```python
from build123d import *

# Parameters (mm, degrees)
EXTRUDE_1_DEPTH          = 25
EXTRUDE_3_DEPTH          = 2.5
EXTRUDE_4_DEPTH          = 2.5
SKETCH_8_R               = 1.5
CUT_EXTRUDE_1_DEPTH      = 31.124740663
SKETCH_9_R               = 1.5
CUT_EXTRUDE_2_DEPTH      = 33.913712948
SKETCH_10_R              = 1.5
CUT_EXTRUDE_3_DEPTH      = 31.745934691
HOLE_WIZARD_2_AT_2_COUNT = 2
HOLE_WIZARD_2_AT_2_PITCH = 8
HOLE_WIZARD_2_AT_3_COUNT = 2
HOLE_WIZARD_2_AT_3_PITCH = 16.124515497
HOLE_WIZARD_2_AT_4_COUNT = 2
HOLE_WIZARD_2_AT_4_PITCH = 14


with BuildPart() as part:
    # 草图1 → 凸台-拉伸1 (new body)
    with BuildSketch(Plane(origin=(0, 0, 0), x_dir=(1, 0, 0), z_dir=(0, 1, 0))):
        Polygon((6, 1.25), (6, 15.75), (8.5, 15.75), (8.5, 1.25), (8.5, -1.25), (-8.5, -1.25), (-8.5, 1.25), align=None)
    extrude(amount=EXTRUDE_1_DEPTH)

    # 草图5 → 凸台-拉伸3 (add)
    with BuildSketch(Plane.XZ):
        Polygon((6, -15.75), (6, -1.25), (-8.5, -1.25), align=None)
    extrude(amount=-EXTRUDE_3_DEPTH)

    # 草图6 → 凸台-拉伸4 (add)
    with BuildSketch(Plane(origin=(0, 25, 0), x_dir=(1, 0, 0), z_dir=(0, 1, 0))):
        Polygon((6, 15.75), (6, 1.25), (-8.5, 1.25), align=None)
    extrude(amount=-EXTRUDE_4_DEPTH)

    # 草图8 → 切除-拉伸1 (cut, through all)
    with BuildSketch(Plane(origin=(0, 0, -1.25), x_dir=(-1, 0, 0), z_dir=(0, 0, -1))):
        with Locations((-2.5, 19.5)):
            Circle(SKETCH_8_R)
        with Locations((5.5, 19.5)):
            Circle(SKETCH_8_R)
        with Locations((5.5, 5.5)):
            Circle(SKETCH_8_R)
        with Locations((-2.5, 5.5)):
            Circle(SKETCH_8_R)
    extrude(amount=-CUT_EXTRUDE_1_DEPTH, mode=Mode.SUBTRACT)

    # 草图9 → 切除-拉伸2 (cut, through all)
    with BuildSketch(Plane.ZY.offset(-6)):
        with Locations((-12.75, 19.5)):
            Circle(SKETCH_9_R)
        with Locations((-12.75, 5.5)):
            Circle(SKETCH_9_R)
        with Locations((-4.75, 19.5)):
            Circle(SKETCH_9_R)
        with Locations((-4.75, 5.5)):
            Circle(SKETCH_9_R)
    extrude(amount=-CUT_EXTRUDE_2_DEPTH, mode=Mode.SUBTRACT)

    # 草图10 → 切除-拉伸3 (cut, through all)
    with BuildSketch(Plane.XZ):
        with Locations(Location((1, -6.25, 0), (0, 0, 270))):
            Circle(SKETCH_10_R)
    extrude(amount=-CUT_EXTRUDE_3_DEPTH, mode=Mode.SUBTRACT)

    # 草图14 → 打孔尺寸(%根据十字)槽沉头木螺钉的类型2 (revolve, cut)
    with BuildSketch(Plane(origin=(-5.5, 5.5, -1.25), x_dir=(0, 1, 0), z_dir=(1, 0, 0))):
        Polygon((0, 0), (0, 2.5), (1.5, 2.5), (1.5, 1.4), (2.9, 0), align=None)
    hole_wizard_2 = revolve(axis=Axis((-5.5, 5.5, -7.6), (0, 0, 1)), mode=Mode.SUBTRACT)

    # 打孔尺寸(%根据十字)槽沉头木螺钉的类型2 at 2: 打孔尺寸(%根据十字)槽沉头木螺钉的类型2 ×2
    with Locations(*[(i * HOLE_WIZARD_2_AT_2_PITCH, 0, 0) for i in range(1, HOLE_WIZARD_2_AT_2_COUNT)]):
        add(hole_wizard_2, mode=Mode.SUBTRACT)

    # 打孔尺寸(%根据十字)槽沉头木螺钉的类型2 at 3: 打孔尺寸(%根据十字)槽沉头木螺钉的类型2 ×2
    with Locations(*[Vector(0.49613893835683387, 0.8682431421244591, 0) * (i * HOLE_WIZARD_2_AT_3_PITCH) for i in range(1, HOLE_WIZARD_2_AT_3_COUNT)]):
        add(hole_wizard_2, mode=Mode.SUBTRACT)

    # 打孔尺寸(%根据十字)槽沉头木螺钉的类型2 at 4: 打孔尺寸(%根据十字)槽沉头木螺钉的类型2 ×2
    with Locations(*[(0, i * HOLE_WIZARD_2_AT_4_PITCH, 0) for i in range(1, HOLE_WIZARD_2_AT_4_COUNT)]):
        add(hole_wizard_2, mode=Mode.SUBTRACT)


solid = part.part
```
Geometry: final body of the model. Coordinates: model frame, mm. A direction names the side the tool comes from. Coordinates: 2 decimals unless noted, no trailing zeros. Order: outer loops, then holes, each group sorted by start corner. A loop starts at its lowest first (then second) coordinate and runs counter-clockwise, first axis right, second up. Notation, with made-up numbers: M -18.75,55 L 32.25,55 A5 ccw 32.25,62 Z; hole C 39.25,-38.5 d9. An arc over 180 degrees is marked long. Answer in a Markdown table with one row per item. Add a question column.
Q1. Section query A-A on y = 5.5. Return the cut outline in (x, z), and give its area (3 significant figures).
Q2. Section query D-D on x = -5.5. Return the cut outline in (y, z).
Q3. Line query: L1, parallel to Y at x = 7.4, z = -12.75; L2, parallel to X at y = 5.5, z = 0.75; L3, parallel to Y at x = -2.25, z = -3.25. Output: solid intervals per line, ascending.
Q4. Reachability of faces 1 (the flat face through (6, 12, -8)), 2 (the cylindrical face through (1.07, 1.23, -4.75)) from +Z, -Z, +X, -X, +Y, -Y: full face, straight path, thin tool, end or side. Return the list, or none.
Q5. Mould query, pull axis Y, two halves, no side actions, for faces 3 (the flat face through (0, 12, 1.25)), 4 (the flat face through (2, 0, -3)), 5 (the flat face through (-1, 12, -1.25)), 6 (the cylindrical face through (-6.93, 5.95, 0.69)). Classes: released by +Y, released by -Y, zero draft, split by the parting line, or undercut.
Q6. Section query B-B on x = 7.5. Return the cut outline in (y, z), and give its area (3 significant figures).
Q7. Contact query for flat-ended pins moving along their axis: P1, Ø1.8, axis at x = -5.5, y = 5.5, coming from the +Z side; P2, Ø4, axis at x = 2.5, y = 19.5, coming from the -Z side; P3, Ø7, axis at y = 8, z = -11.5, coming from the -X side; P4, Ø8, axis at x = -6.5, y = 13, coming from the -Z side. Output: stop coordinate, or through.
Q8. Section query C-C on z = -12.75. Return the cut outline in (x, y), and give its area (3 significant figures).
Completed:
| question | item | result |
|---|---|---|
| 1 | outline | M -8.5,-1.25 L -8.4,-1.25 L -7,0.15 L -7,1.25 L -8.5,1.25 Z; M -4,0.15 L -2.6,-1.25 L -0.4,-1.25 L 1,0.15 L 1,1.25 L -4,1.25 Z; M 4,0.15 L 5.4,-1.25 L 6,-1.25 L 6,-3.25 L 8.5,-3.25 L 8.5,1.25 L 4,1.25 Z; M 6,-15.75 L 8.5,-15.75 L 8.5,-14.25 L 6,-14.25 Z; M 6,-11.25 L 8.5,-11.25 L 8.5,-6.25 L 6,-6.25 Z |
| 1 | area | 44.8 mm2 |
| 2 | outline | M 0,-4.25 L 2.5,-4.25 L 2.5,-1.25 L 2.6,-1.25 L 4,0.15 L 4,1.25 L 0,1.25 Z; M 7,0.15 L 8.4,-1.25 L 16.6,-1.25 L 18,0.15 L 18,1.25 L 7,1.25 Z; M 21,0.15 L 22.4,-1.25 L 22.5,-1.25 L 22.5,-4.25 L 25,-4.25 L 25,1.25 L 21,1.25 Z |
| 3 | L1 | y = 0 to 4, 7 to 18, 21 to 25 |
| 3 | L2 | x = -8.5 to -7, -4 to 1, 4 to 8.5 |
| 3 | L3 | y = 0 to 2.5, 22.5 to 25 |
| 4 | face 1 | -Z, -X |
| 4 | face 2 | +Y, -Y |
| 5 | face 3 | zero draft |
| 5 | face 4 | released by -Y |
| 5 | face 5 | undercut |
| 5 | face 6 | undercut |
| 6 | outline | M 0,-15.75 L 25,-15.75 L 25,1.25 L 0,1.25 Z; hole C 5.5,-12.75 d3; hole C 5.5,-4.75 d3; hole C 19.5,-12.75 d3; hole C 19.5,-4.75 d3 |
| 6 | area | 397 mm2 |
| 7 | P1 | passes through |
| 7 | P2 | stops at z = -0.35 |
| 7 | P3 | stops at x = 6 |
| 7 | P4 | stops at z = -1.25 |
| 8 | outline | M 3,0 L 8.5,0 L 8.5,4 L 6,4 L 6,2.5 L 3,2.5 Z; M 3,22.5 L 6,22.5 L 6,21 L 8.5,21 L 8.5,25 L 3,25 Z; M 6,7 L 8.5,7 L 8.5,18 L 6,18 Z |
| 8 | area | 62.5 mm2 |
